Autodesk Inventor part; units mm, degrees
ref_plane "YZ Plane" through (0, 0, 0) normal (1, 0, 0) x (0, 1, 0)
ref_plane "XZ Plane" through (0, 0, 0) normal (0, 1, 0) x (-1, 0, 0)
ref_plane "XY Plane" through (0, 0, 0) normal (0, 0, 1) x (1, 0, 0)
sketch "Sketch1" plane through (0, 0, 0) normal (0, 1, 0) x (-1, 0, 0)
  line L0 (29, 24.5) -> (-29, 24.5) construction
  line L1 (-29, 24.5) -> (-29, -24.5) construction
  line L2 (-29, -24.5) -> (29, -24.5) construction
  line L3 (29, -24.5) -> (29, 24.5) construction
  circle A0 centre (29, 24.5) radius 3
  circle A1 centre (29, -24.5) radius 3
  circle A2 centre (-29, -24.5) radius 3
  circle A3 centre (-29, 24.5) radius 3
  point P0 (0, 0)
  dimension "d0" = 24.5
  dimension "d1" = 29
  dimension "d2" = 58
  dimension "d3" = 49
  dimension "d4" = 6
  dimension "d5" = 6
  dimension "d6" = 6
  dimension "d7" = 6
extrude "Extrusion1" add sketch "Sketch1" along normal blind 5
sketch "Sketch6" plane through (0, 0, 0) normal (0, 1, 0) x (-1, 0, 0)
  line L0 (33.8, -29.3) -> (-55, -29.3)
  line L1 (-55, -29.3) -> (-55, 29.3)
  line L2 (-55, 29.3) -> (33.8, 29.3)
  line L3 (33.8, 29.3) -> (33.8, -29.3)
  circle A0 centre (29, -24.5) radius 3
  circle A1 centre (-29, 24.5) radius 3
  circle A2 centre (29, 24.5) radius 3
  circle A3 centre (-29, -24.5) radius 3
  line L4 (32, -27.5) -> (-32, -27.5)
  line L5 (-32, -27.5) -> (-32, 27.5)
  line L6 (-32, 27.5) -> (32, 27.5)
  line L7 (32, 27.5) -> (32, -27.5)
  point P0 (0, 0)
  dimension "d30" = 1.8
  dimension "d31" = 55
  dimension "d32" = 64
  dimension "d33" = 27.5
  dimension "d34" = 32
  dimension "d35" = 1.8
  dimension "d36" = 1.8
  dimension "d37" = 23
extrude "Extrusion5" add sketch "Sketch6" against normal blind 3 contours L0 L1 L2 L3 | A0 | L7 L4 A0 | A0 L4 A3 L5 A1 L6 A2 L7 | A2 | A2 L6 L7 | L4 L5 A3 | A3 | A1 | A1 L5 L6
fillet "Fillet2" radius 2 4 edges at (-33.8, -1.5, 29.3) (55, -1.5, 29.3) (55, -1.5, -29.3) (-33.8, -1.5, -29.3)
sketch "Sketch7" plane through (0, 0, 0) normal (0, 1, 0) x (1, 0, 0)
  circle A0 centre (29, 24.5) radius 3
  circle A1 centre (-29, 24.5) radius 3
  circle A2 centre (29, -24.5) radius 3
  circle A3 centre (-29, -24.5) radius 3
  arc A4 (-31.8, 29.3) -> (-33.8, 27.3) centre (-31.8, 27.3) ccw
  line L0 (-33.8, 27.3) -> (-33.8, -27.3)
  arc A5 (-33.8, -27.3) -> (-31.8, -29.3) centre (-31.8, -27.3) ccw
  line L1 (-31.8, -29.3) -> (53, -29.3)
  arc A6 (53, -29.3) -> (55, -27.3) centre (53, -27.3) ccw
  line L2 (55, -27.3) -> (55, 27.3)
  arc A7 (55, 27.3) -> (53, 29.3) centre (53, 27.3) ccw
  line L3 (53, 29.3) -> (-31.8, 29.3)
  line L4 (53.8, 27.3) -> (53.8, -27.3)
  arc A8 (53, -28.1) -> (53.8, -27.3) centre (53, -27.3) ccw
  line L5 (53, -28.1) -> (-31.8, -28.1)
  arc A9 (-32.6, -27.3) -> (-31.8, -28.1) centre (-31.8, -27.3) ccw
  line L6 (-32.6, -27.3) -> (-32.6, 27.3)
  arc A10 (-31.8, 28.1) -> (-32.6, 27.3) centre (-31.8, 27.3) ccw
  line L7 (-31.8, 28.1) -> (53, 28.1)
  arc A11 (53.8, 27.3) -> (53, 28.1) centre (53, 27.3) ccw
  point P0 (0, 0)
  dimension "d41" = 1.2
extrude "Extrusion6" add sketch "Sketch7" along normal blind 6.5 contours L3 A7 L2 A6 L1 A5 L0 A4
sketch "Sketch8" plane through (0, 0, 0) normal (0, 1, 0) x (1, 0, 0)
  arc A0 (-31.8, 28.1) -> (-32.6, 27.3) centre (-31.8, 27.3) ccw
  line L0 (-32.6, 27.3) -> (-32.6, -27.3)
  arc A1 (-32.6, -27.3) -> (-31.8, -28.1) centre (-31.8, -27.3) ccw
  line L1 (-31.8, -28.1) -> (53, -28.1)
  arc A2 (53, -28.1) -> (53.8, -27.3) centre (53, -27.3) ccw
  line L2 (53.8, -27.3) -> (53.8, 27.3)
  arc A3 (53.8, 27.3) -> (53, 28.1) centre (53, 27.3) ccw
  line L3 (53, 28.1) -> (-31.8, 28.1)
  circle A4 centre (29, 24.5) radius 3
  circle A5 centre (-29, 24.5) radius 3
  circle A6 centre (29, -24.5) radius 3
  circle A7 centre (-29, -24.5) radius 3
  circle A8 centre (-29, -24.5) radius 3
  line L4 (-29, -21.5) -> (-32.6, -21.5)
  line L5 (-32.6, 27.3) -> (-32.6, -27.3)
  line L6 (-26, -24.5) -> (-26, -28.1)
  line L7 (-31.8, -28.1) -> (53, -28.1)
  circle A9 centre (-29, 24.5) radius 3
  line L8 (-29, 21.5) -> (-32.6, 21.5)
  line L9 (-26, 24.5) -> (-26, 28.1)
  line L10 (53, 28.1) -> (-31.8, 28.1)
  circle A10 centre (29, 24.5) radius 3
  line L11 (26, 24.5) -> (26, 28.1)
  line L12 (32, 24.5) -> (32, 28.1)
  circle A11 centre (29, -24.5) radius 3
  line L13 (32, -24.5) -> (32, -28.1)
  line L14 (26, -24.5) -> (26, -28.1)
  point P0 (0, 0)
extrude "Extrusion7" add sketch "Sketch8" along normal blind 4.8 contours L3 L9 A5 L8 L0 A0 | L3 L12 A4 L11 | L4 A7 L6 L1 A1 L0 | L14 A6 L13 L1
sketch "Sketch9" plane through (-33.8, -3, -27.3) normal (-1, 0, 0) x (0, 0, 1)
  line L0 (0, 0) -> (0, 9.5)
  line L1 (54.6, 0) -> (0, 0)
  line L2 (54.6, 9.5) -> (54.6, 0)
  line L3 (0, 9.5) -> (54.6, 9.5)
  line L4 (19.8, 14.5) -> (34.8, 14.5)
  line L5 (34.8, 14.5) -> (34.8, 4.5)
  line L6 (34.8, 4.5) -> (19.8, 4.5)
  line L7 (19.8, 4.5) -> (19.8, 14.5)
  line L8 (0, 9.5) -> (54.6, 9.5)
  line L9 (19.8, 14.5) -> (34.8, 4.5) construction
  line L10 (34.8, 14.5) -> (19.8, 4.5) construction
  point P0 (27.3, 3)
  point P1 (27.3, 9.5)
  point P2 (34.8, 9.5)
  point P3 (19.8, 9.5)
  dimension "d46" = 15
  dimension "d47" = 10
extrude "Extrusion8" cut sketch "Sketch9" against normal up to next contours L3 L5 L6 L7
sketch "Sketch10" plane through (-29, 5, 24.5) normal (0, 1, 0) x (1, 0, 0)
  circle A0 centre (0, 0) radius 3
  circle A1 centre (0, 49) radius 3
  circle A2 centre (58, 49) radius 3
  circle A3 centre (58, 0) radius 3
  point P0 (29, 24.5)
hole "Hole2" at (-29, 5, 24.5) at (-29, 5, -24.5) at (29, 5, -24.5) at (29, 5, 24.5) direction (0, -1, 0) diameter 3.3 end through all
properties part number "Pi Back Mount"
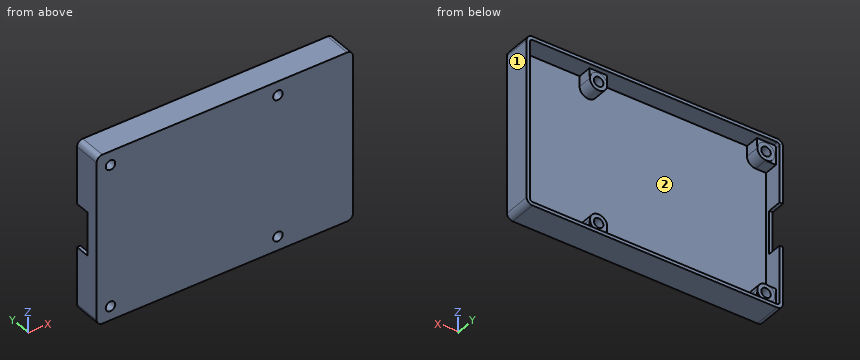
Can you work these out from the model? Positions are in its coordinate system, mm. Face numbers are marked on the shaded views. A direction names the side the tool comes from. Coordinates: 2 decimals unless noted, no trailing zeros. Order: outer loops, then holes, each group sorted by start corner. A loop starts at its lowest first (then second) coordinate and runs counter-clockwise, first axis right, second up. Notation, with made-up numbers: (-19.75, -2) -> (5.25, -2) arc R24 cw to (5.25, 13) -> close; hole circle Ø6 at (30, -34.5). An arc over 180 degrees is marked (long way). Use one line per item in the form item = value.
Q1. I need wall thicknesses on L1, parallel to Z at x = 29, y = 3; L2, parallel to Z at x = -29, y = -1.5; L3, parallel to X at y = -0.5, z = 24.5. Which ranges of each line are inside material? Lowest first, please.
From the geometry:
L1 = -29.3 to -26.15, -22.85 to -21.5, 21.5 to 22.85, 26.15 to 29.3
L2 = -29.3 to -26.15, -22.85 to 22.85, 26.15 to 29.3
L3 = -33.8 to -30.65, -27.35 to 27.35, 30.65 to 55
Q2. Will these pins go through, and if not, where does the flat tip stop? P1, Ø5.5, axis at x = 29, z = -24.5, coming from the +Y side; P2, Ø1.3, axis at x = -33, y = 3, coming from the -Z side; P3, Ø1.3, axis at x = -33.5, y = 3.5, coming from the +Z side.
From the geometry:
P1 = 5
P2 = -29.22
P3 = 29
Q3. Imagine slicing it at A-A, the plane z = -4. List the corners of the cut face in (x, y) for me, then the cut area to 3 significant figures.
From the geometry:
outline = (-33.8, -3) -> (55, -3) -> (55, 6.5) -> (53.8, 6.5) -> (53.8, 0) -> (-32.6, 0) -> (-32.6, 1.5) -> (-33.8, 1.5) -> close
area = 276 mm²
Q4. Which directions (+Z, -Z, +X, -X, +Y, -Y) give clear straight access to the entire face, cutting with the end or side of a thin tool? Please do the marked faces 1 and 2.
From the geometry:
face_1 = +Z, -Z, +X, +Y, -Y
face_2 = +Y
Q5. Imagine slicing it at B-B, the plane x = -25. List the corners of the cut face in (y, z) for me.
From the geometry:
outline = (-3, -29.3) -> (6.5, -29.3) -> (6.5, -28.1) -> (0, -28.1) -> (0, 28.1) -> (6.5, 28.1) -> (6.5, 29.3) -> (-3, 29.3) -> close
